Source: CAD feature listing. Evaluate the final solid. Frame: model axes, mm. A direction names the side the tool comes from. Coordinates: 2 decimals unless noted, no trailing zeros. Write each loop counter-clockwise with the first axis right and the second up, starting at its lowest first coordinate (ties: lowest second). Pieces come first, ordered by that corner, then holes. Notation, with made-up numbers: M 25.5,78 L 45.5,78 A5 ccw 45.5,84 Z; hole C -36.75,-19.75 d8. An arc over 180 degrees is marked long. Answer as CSV lines item,"result". Start each with the question number.
1. Section B-B on x = 19.5. Return the cut outline in (y, z).
2. Line query: probe 1 along Y at (x, z) = (0, 1.3); probe 2 along Y at (x, z) = (8, 0.6); probe 3 along X at (y, z) = (-42, 4.25). Output: solid intervals per line, ascending. Write a range as [from, to].
3. Section A-A on z = 1.35. Return the cut outline in (x, y).
4. Reachability of faces 4 (the face through (69.343, -43.594, 2.465)), 5 (the face through (69.492, -29.836, 2.465)), 6 (the face through (73.1, -33.9, 2.5)) from +Z, -Z, +X, -X, +Y, -Y: full face, straight path, thin tool, end or side. Return the list, or none.
5. Mould query, pull axis Y, two halves, no side actions, for faces 1 (the face through (62.833, -9.287, 2.465)), 2 (the face through (41.073, -53.277, 2.465)), 3 (the face through (71.31, -39.02, 2.46)). Classes: pulls with the +Y half, pulls with the -Y half, needs draft (parallel to the pull), parting line crosses it, or undercut.
6. Contact query for flat-ended pins moving along their axis: pin 1 Ø1.5 at (x, z) = (-14, 2.5) entering from +Y; pin 2 Ø3 at (x, z) = (22, 0.5) entering from -Y; pin 3 Ø3 at (x, z) = (-35, 4) entering from -Y. Output: stop coordinate, or through.
7. Section C-C on y = 7. Return the cut outline in (x, z).
```python
from build123d import *

# Parameters (mm, degrees)
BOSS_EXTRUDE1_DEPTH = 5


with BuildPart() as part:
    # Sketch1 → Boss-Extrude1 (new body)
    with BuildSketch(Plane.XY):
        with BuildLine():
            Line((58.948050608, 11.186032786), (66.828328123, -30.341379713))
            Line((66.828328123, -30.341379713), (72.231899429, -29.315993374))
            Line((72.231899429, -29.315993374), (73.977656704, -38.515768682))
            Line((73.977656704, -38.515768682), (68.574085398, -39.541155021))
            Line((68.574085398, -39.541155021), (70.134083395, -47.762017822))
            Line((70.134083395, -47.762017822), (11.186032786, -58.948050608))
            ThreePointArc((11.186032786, -58.948050608), (-49.592285961, 33.772846685), (58.948050608, 11.186032786))
        make_face()
    extrude(amount=BOSS_EXTRUDE1_DEPTH)


solid = part.part
```
Values:
1,outline,"M -57.37,0 L 56.74,0 L 56.74,5 L -57.37,5 Z"
2,probe 1,"[-60, 60]"
2,probe 2,"[-59.46, 59.46]"
2,probe 3,"[-42.85, 69.04]"
3,outline,"M 11.19,-58.95 L 70.13,-47.76 L 68.57,-39.54 L 73.98,-38.52 L 72.23,-29.32 L 66.83,-30.34 L 58.95,11.19 A60 ccw long Z"
4,face 4,"+Z, -Z, +X"
4,face 5,"+Z, -Z, +Y"
4,face 6,"+Z, -Z, +X, +Y"
5,face 1,"pulls with the +Y half"
5,face 2,"pulls with the -Y half"
5,face 3,"undercut"
6,pin 1,"y = 58.52"
6,pin 2,"y = -57.18"
6,pin 3,"y = -49.78"
7,outline,"M -59.59,0 L 59.74,0 L 59.74,5 L -59.59,5 Z"
